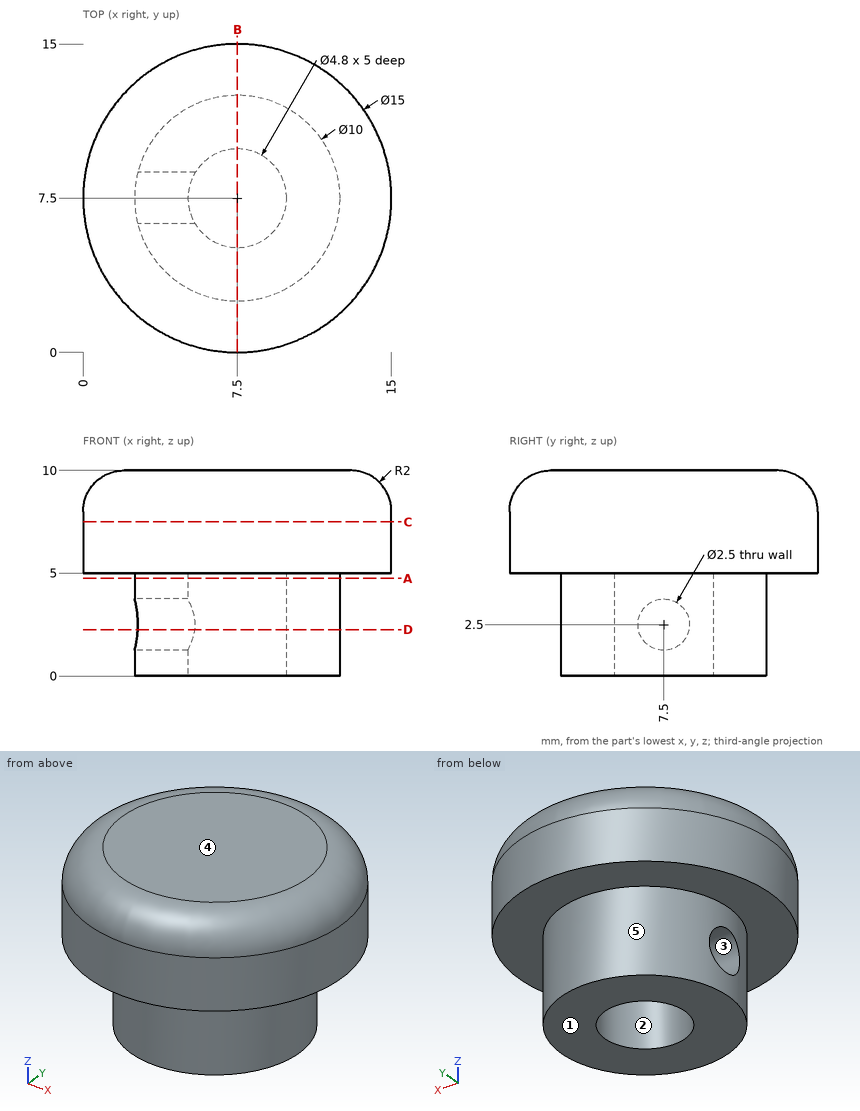
For this review, use the dimensioned drawing (mm, ordinates from the lowest corner) and the shaded views. A direction names the side the tool comes from. Round coordinates to 2 decimals unless told otherwise and drop trailing zeros. Write each loop counter-clockwise with the first axis right and the second up, starting at its lowest first coordinate (ties: lowest second). Pieces come first, ordered by that corner, then holes. Notation, with made-up numbers: (30.25, 46) - (73.25, 46) arc R26 ccw to (73.25, 76) - close; hole circle Ø3 at (75, 4.5). An arc over 180 degrees is marked (long way). One line per item, written item: value. Start each with the question number.
1. Machinability: for the marked faces 1 and 2, which of the approach directions +Z, -Z, +X, -X, +Y, -Y give a long, thin tool a straight path to every point of the face, cutting with its end or side? Answer none if there is none.
2. Consider section D-D on z = 2.25. Write out the cut boundary in (x, y), and give its area (3 significant figures).
3. Clearance check with flat-ended pins moving along their axes: P1, Ø5, axis at x = 5, z = 8.5, coming from the -Y side; P2, Ø2, axis at x = 10, z = 7, coming from the +Y side; P3, Ø3, axis at y = 7.5, z = 2.5, coming from the +X side; P4, Ø1, axis at x = 3.5, z = 3.5, coming from the +Y side. State where each tip first meets the part, or that it passes through.
4. The part is to be moulded in two halves that separate along Y. For the marked faces 3, 4 and 5, say which applies: released by +Y, released by -Y, zero draft, split by the parting line, or undercut.
5. Consider section C-C on z = 7.5. Write out the cut boundary in (x, y).
6. Consider section B-B on x = 7.5. Write out the cut boundary in (y, z), and give its area (3 significant figures).
7. To check wall thickness, follow L1, parallel to Z at x = 2.5, y = 6.75; L2, parallel to Y at x = 4.35, z = 2.5; L3, parallel to Y at x = 4.6, z = 2.5. State the ranges of each line that lie inside material, in increasing order. Write a range as from..to.
8. Consider section A-A on z = 4.75. Write out the cut boundary in (x, y).
Checks:
1. face 1: -Z, +X, -X, +Y, -Y
1. face 2: -Z
2. outline: (2.65, 6.28) arc R5 ccw (long way) to (2.65, 8.72) - (5.44, 8.72) arc R2.4 cw (long way) to (5.44, 6.28) - close
2. area: 53.9 mm^2
3. P1: stops at y = 0
3. P2: stops at y = 14.85
3. P3: stops at x = 12.5
3. P4: stops at y = 11.07
4. face 3: undercut
4. face 4: zero draft
4. face 5: split by the parting line
5. outline: circle Ø15 at (7.5, 7.5)
6. outline: (0, 5) - (2.5, 5) - (2.5, 0) - (5.1, 0) - (5.1, 5) - (9.9, 5) - (9.9, 0) - (12.5, 0) - (12.5, 5) - (15, 5) - (15, 8) arc R2 ccw to (13, 10) - (2, 10) arc R2 ccw to (0, 8) - close
6. area: 99.3 mm^2
7. L1: z = 5..10
7. L2: y = 3.62..6.25, 8.75..11.38
7. L3: y = 3.43..6.25, 8.75..11.57
8. outline: circle Ø10 at (7.5, 7.5); hole circle Ø4.8 at (7.5, 7.5)
